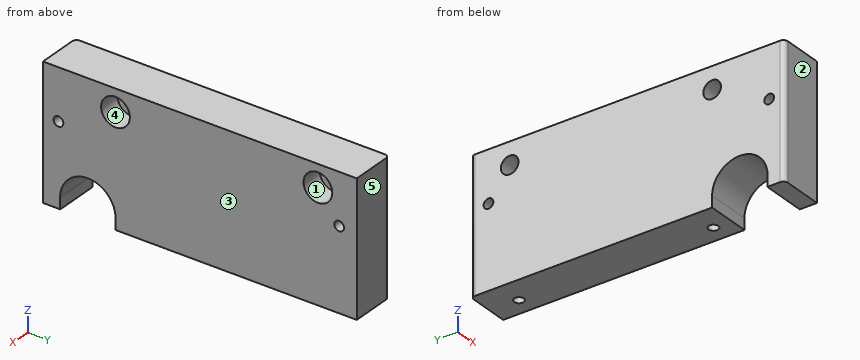
from build123d import *

# Parameters (mm, degrees)
F0_W           = 90.17
F0_H           = 38.1
F1_DEPTH       = 12.7
F2_D           = 2.794
F4_D           = 5.08
F4_CBORE_D     = 8.255
F4_CBORE_DEPTH = 6.35
F6_DEPTH       = 12.701
F8_D           = 2.794
F8_DEPTH       = 25.4
F8_TIP         = 0.8394022848
F9_R           = 1.27


with BuildPart() as f1:
    # F0 (on Right) → F1 (new body)
    with BuildSketch(Plane.YZ):
        with Locations((19.7381743398, -3.2925931737)):
            Rectangle(F0_W, F0_H)
    extrude(amount=F1_DEPTH)

    # F2 (through all)
    with Locations(Plane(origin=(0, 0, 0), x_dir=(0, 1, 0), z_dir=(-1, 0, 0))):
        with Locations((-20.9018256602, -1.1524068263), (59.7431743398, -1.1524068263)):
            Hole(F2_D / 2)

    # F4 (through all)
    with Locations(Plane.YZ.offset(12.7)):
        with Locations((-4.5188256602, 9.4074068263), (53.6471743398, 9.4074068263)):
            CounterBoreHole(F4_D / 2, F4_CBORE_D / 2, F4_CBORE_DEPTH)

    # F5 (on Right) → F6 (cut, through all)
    with BuildSketch(Plane.YZ):
        with BuildLine():
            ThreePointArc((-4.5006518298, -19.1675931737), (-12.3808319272, -11.1898662261), (-20.4548983074, -18.9713068193))
            ThreePointArc((-20.4548983074, -18.9713068193), (-20.4573256602, -19.1675931737), (-20.4548983074, -19.3638795281))
            Line((-20.4548983074, -19.3638795281), (-20.3756518298, -22.5674978264))
            Line((-20.3756518298, -22.5674978264), (-4.5006518298, -22.5674978264))
            Line((-4.5006518298, -22.5674978264), (-4.5006518298, -19.1675931737))
        make_face()
    extrude(amount=F6_DEPTH, mode=Mode.SUBTRACT)

    # F8
    with Locations(Plane(origin=(0, 0, -22.3425931737), x_dir=(1, 0, 0), z_dir=(0, 0, -1))):
        with Locations((7.62, -0.6881743398), (7.62, -56.5681743398)):
            Hole(F8_D / 2, depth=F8_DEPTH)
            with Locations((0, 0, -(F8_DEPTH + F8_TIP / 2))):  # 118° drill point
                Cone(0, F8_D / 2, F8_TIP, mode=Mode.SUBTRACT)

    # F9
    f9_edges = [f1.edges().sort_by_distance(p)[0] for p in [
        (0, -25.346826, -3.292593),
        (0, 64.823174, -3.292593),
    ]]
    fillet(f9_edges, radius=F9_R)


solid = f1.part
The listing builds one solid part. Answer for the finished solid, in the listing's coordinates (mm). Face numbers are marked on the shaded views. A direction names the side the tool comes from. Round coordinates to 2 decimals unless told otherwise and drop trailing zeros. Write each loop counter-clockwise with the first axis right and the second up, starting at its lowest first coordinate (ties: lowest second). Pieces come first, ordered by that corner, then holes. Notation, with made-up numbers: (-9, 2.5) - (35, 2.5) arc R23 ccw to (35, 39.5) - close; hole circle Ø1 at (32.5, -31.75). An arc over 180 degrees is marked (long way). Use a Markdown table: item, result. Add a question column.
1. Flat-ended cylindrical pins translate along their axes: P1, Ø6.5, axis at y = -4.52, z = 9.41, coming from the +X side; P2, Ø2, axis at x = 7.62, y = 56.57, coming from the -Z side. Find the tip coordinate at first contact, or state that the pin passes through.
2. For a pull along Y with two mould halves and no side action, classify the marked faces 1, 2 and 3 as +Y half, -Y half, draft (parallel to the pull), parting line (faces both ways), or undercut.
3. A tool of negligible diameter and unlimited length cuts with its end or side. For the marked faces 4 and 5, from which of +Z, -Z, +X, -X, +Y, -Y can it reach the whole face along a straight path? Write none if from no direction.
4. The part is cut by section A-A (z = -15.5). Write down the section's boundary in (x, y).
5. Consider line 1 (Z direction, x = 1.25, y = -21); line 2 (Y direction, x = 10.25, z = 11.5); line 3 (Y direction, x = 6.75, z = -1). Determine where each line is inside the solid, lowest interval first.
Reported:
| question | item | result |
|---|---|---|
| 1 | P1 | x = 6.35 |
| 1 | P2 | z = 3.29 |
| 2 | face 1 | undercut |
| 2 | face 2 | -Y half |
| 2 | face 3 | draft |
| 3 | face 4 | +X |
| 3 | face 5 | +Z, -Z, +X, -X, +Y |
| 4 | outline | (0, -24.08) arc R1.27 ccw to (1.27, -25.35) - (12.7, -25.35) - (12.7, -19.56) - (0, -19.56) - close; (0, -5.39) - (12.7, -5.39) - (12.7, 64.82) - (1.27, 64.82) arc R1.27 ccw to (0, 63.55) - close; hole circle Ø2.79 at (7.62, 0.69); hole circle Ø2.79 at (7.62, 56.57) |
| 5 | line 1 | -22.34 to -0.24, 2.55 to 15.76 |
| 5 | line 2 | -25.35 to -8.08, -0.96 to 50.09, 57.2 to 64.82 |
| 5 | line 3 | -25.35 to -0.4, 1.78 to 55.48, 57.66 to 64.82 |
